Check sheet for the drawn part. Datum: minimum x, y, z corner. Units: mm. Coordinates: 2 decimals unless noted, no trailing zeros. Order: outer loops, then holes, each group sorted by start corner. A loop starts at its lowest first (then second) coordinate and runs counter-clockwise, first axis right, second up. Notation, with made-up numbers: (-14.5, -21) - (39.5, -21) arc R26 cw to (39.5, 9) - close; hole circle Ø11 at (8, 39). An arc over 180 degrees is marked (long way). Return JSON: item names as keys, results as strings. Group by question number.
Item 1: Section check A-A on z = 19.5. Enter the section's corners in (x, y), then the cut area to 3 significant figures.
Item 2: Scan lines: probe 1 along X at (y, z) = (2.6, 11); probe 2 along Z at (x, y) = (7.5, 2.1); probe 3 along Z at (x, y) = (31.5, 2.6). Record each from-to range of solid material in increasing order.
Item 3: Gauge pin test, flat ends, axial feed: pin 1 (0.8 mm diameter, centred on x = 0.5, z = 17.5, fed in from +Y); pin 2 (1.6 mm diameter, centred on y = 2.5, z = 20, fed in from +X); pin 3 (0.6 mm diameter, centred on y = 2.5, z = 31, fed in from -X). Record the tip position at first contact, or that the pin passes through.
Item 4: Section check B-B on y = 1.45. Enter the section's corners in (x, z).
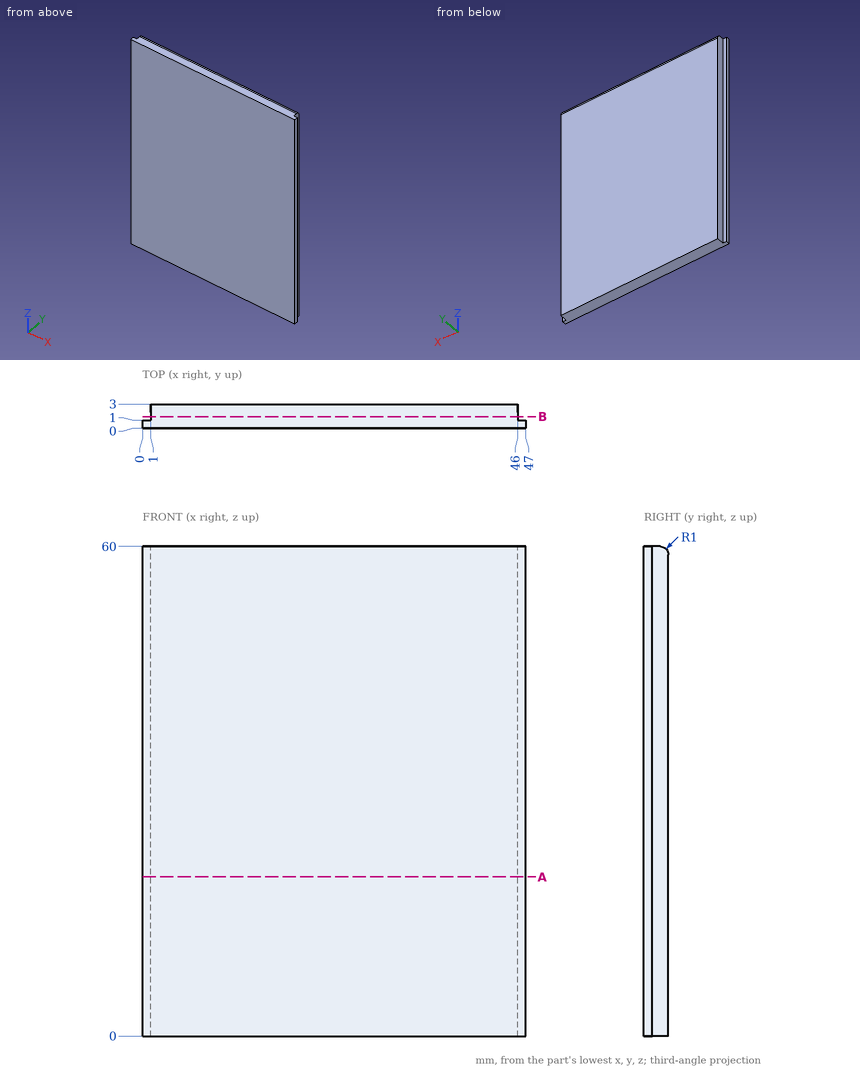
Computed:
{
 "1": {"outline": "(0, 0) - (47, 0) - (47, 1) - (46, 1) - (46, 3) - (1, 3) - (1, 1) - (0, 1) - close", "area": "137 mm²"},
 "2": {"probe 1": "x = 1 to 46", "probe 2": "z = 0 to 59.99", "probe 3": "z = 0 to 59.8"},
 "3": {"pin 1": "stops at y = 1", "pin 2": "stops at x = 46", "pin 3": "stops at x = 1"},
 "4": {"outline": "(1, 0) - (46, 0) - (46, 60) - (1, 60) - close"}
}
